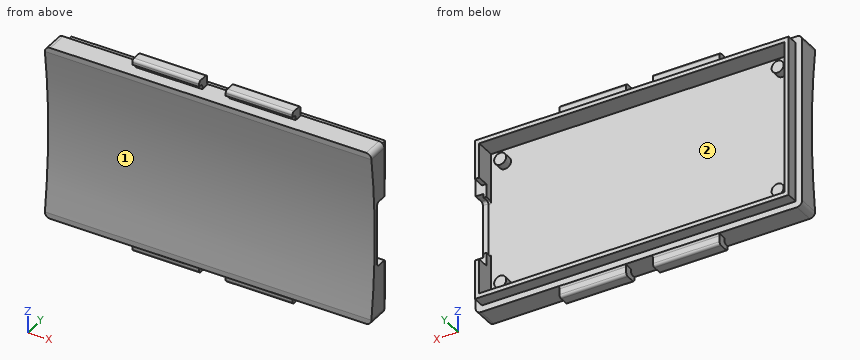
from build123d import *

# Parameters (mm, degrees)
SKETCH2_W               = 61.2
SKETCH2_H               = 32.7
BOSS_EXTRUDE1_DEPTH     = 1.5
BOSS_EXTRUDE2_START     = 1.5
SKETCH2_3_R             = 1.125
BOSS_EXTRUDE2_DEPTH     = 1.5
SKETCH2_7_W             = 61.2
SKETCH2_7_H             = 32.7
BOSS_EXTRUDE5_DEPTH     = 1
FILLET1_R               = 1
CUT_EXTRUDE2_DEPTH      = 35.823591142
CUT_EXTRUDE2_DEPTH_BACK = 0.75
CUT_EXTRUDE2_START      = 1.5
SKETCH2_5_W             = 1.5
SKETCH2_5_H             = 0.75
SKETCH2_5_H_2           = 10.7
FILLET3_R               = 0.5
BOSS_EXTRUDE4_DEPTH     = 2.2
BOSS_EXTRUDE6_DEPTH     = 15
CUT_EXTRUDE4_DEPTH      = 2.5
FILLET4_R               = 0.5
FILLET4_OF_MIRROR1_R    = 0.5
FILLET5_R               = 0.5
CUT_EXTRUDE5_DEPTH      = 37.057211484
CUT_EXTRUDE5_DEPTH_BACK = 37.057211484


with BuildPart() as part:
    # Sketch2 → Boss-Extrude1 (new body)
    with BuildSketch(Plane(origin=(0, 0, 0), x_dir=(1, 0, 0), z_dir=(0, 1, 0))):
        Rectangle(SKETCH2_W, SKETCH2_H)
    extrude(amount=BOSS_EXTRUDE1_DEPTH)

    # Sketch2<3> → Boss-Extrude2 (add)
    with BuildSketch(Plane(origin=(0, 0, 0), x_dir=(1, 0, 0), z_dir=(0, 1, 0)).offset(BOSS_EXTRUDE2_START)):
        Polygon((-30.6, 16.35), (-30.6, -16.35), (30.6, -16.35), (30.6, -6.1), (29.1, -6.1), (29.1, -5.35), (28.6, -5.35), (28.6, -14.35), (-28.6, -14.35), (-28.6, 14.35), (28.6, 14.35), (28.6, 5.35), (30.6, 5.35), (30.6, 16.35), align=None)
        with Locations(Location((-26, 11.75, 0), (0, 0, 270))):
            Circle(SKETCH2_3_R)
        with Locations(Location((-26, -11.75, 0), (0, 0, 270))):
            Circle(SKETCH2_3_R)
        with Locations(Location((26, -11.75, 0), (0, 0, 270))):
            Circle(SKETCH2_3_R)
        with Locations(Location((26, 11.75, 0), (0, 0, 270))):
            Circle(SKETCH2_3_R)
    extrude(amount=BOSS_EXTRUDE2_DEPTH)

    # Sketch2<7> → Boss-Extrude5 (add)
    with BuildSketch(Plane(origin=(0, 0, 0), x_dir=(1, 0, 0), z_dir=(0, 1, 0))):
        Rectangle(SKETCH2_7_W, SKETCH2_7_H)
    extrude(amount=-BOSS_EXTRUDE5_DEPTH)

    # Fillet1
    fillet1_edges = [part.edges().sort_by_distance(p)[0] for p in [
        (-30.6, 1, -16.35),
        (30.6, 1, -16.35),
        (30.6, 1, 16.35),
        (-30.6, 1, 16.35),
    ]]
    fillet(fillet1_edges, radius=FILLET1_R)

    # Sketch2<5> → Cut-Extrude2 (cut, two sides: drawn at the far end of the back side and taken through both)
    with BuildSketch(Plane(origin=(0, 0, 0), x_dir=(1, 0, 0), z_dir=(0, 1, 0)).offset(CUT_EXTRUDE2_START - CUT_EXTRUDE2_DEPTH_BACK)):
        with Locations((29.85, 5.725)):
            Rectangle(SKETCH2_5_W, SKETCH2_5_H)
        with Locations((29.85, 0)):
            Rectangle(SKETCH2_5_W, SKETCH2_5_H_2)
        with Locations((29.85, -5.725)):
            Rectangle(SKETCH2_5_W, SKETCH2_5_H)
    extrude(amount=CUT_EXTRUDE2_DEPTH + CUT_EXTRUDE2_DEPTH_BACK, mode=Mode.SUBTRACT)

    # Fillet3
    fillet3_edges = [part.edges().sort_by_distance(p)[0] for p in [
        (29.85, 0.75, 6.1),
        (29.85, 0.75, -6.1),
        (28.85, 1.5, -5.35),
        (28.85, 1.5, 5.35),
    ]]
    fillet(fillet3_edges, radius=FILLET3_R)

    # Sketch4 → Boss-Extrude4 (add)
    with BuildSketch(Plane(origin=(0, 3, 0), x_dir=(1, 0, 0), z_dir=(0, 1, 0))):
        Polygon((29.4, 15.15), (-29.4, 15.15), (-29.4, -15.15), (29.4, -15.15), (29.4, -7.8), (28.6, -7.8), (28.6, -14.35), (-28.6, -14.35), (-28.6, 14.35), (28.6, 14.35), (28.6, 7.8), (29.4, 7.8), align=None)
    extrude(amount=BOSS_EXTRUDE4_DEPTH)

    # Sketch5 → Boss-Extrude6 (add, symmetric)
    with BuildSketch(Plane(origin=(0, 0, 0), x_dir=(0, 0, -1), z_dir=(1, 0, 0))):
        Polygon((-16.35, 2.8), (-18.35, 2.8), (-18.35, 0.3), (-17.35, 0.3), (-17.35, 1.3), (-16.35, 1.3), align=None)
    boss_extrude6 = extrude(amount=BOSS_EXTRUDE6_DEPTH, both=True)

    # Sketch5<3> → Cut-Extrude4 (cut, symmetric)
    with BuildSketch(Plane(origin=(0, 0, 0), x_dir=(0, 0, -1), z_dir=(1, 0, 0))):
        Polygon((-16.35, 2.8), (-18.35, 2.8), (-18.35, 0.3), (-17.35, 0.3), (-17.35, 1.3), (-16.35, 1.3), align=None)
    cut_extrude4 = extrude(amount=CUT_EXTRUDE4_DEPTH, both=True, mode=Mode.SUBTRACT)

    # Fillet4
    fillet4_edges = [part.edges().sort_by_distance(p)[0] for p in [
        (8.75, 1.3, 17.35),
        (8.75, 2.8, 18.35),
        (8.75, 0.3, 18.35),
        (-8.75, 0.3, 18.35),
        (-8.75, 2.8, 18.35),
        (-8.75, 1.3, 17.35),
    ]]
    fillet(fillet4_edges, radius=FILLET4_R)

    # Mirror1: Boss-Extrude6, Cut-Extrude4 across plane
    add(boss_extrude6.mirror(Plane.XY))
    add(cut_extrude4.mirror(Plane.XY), mode=Mode.SUBTRACT)

    # Fillet4 of Mirror1
    fillet4_of_mirror1_edges = [part.edges().sort_by_distance(p)[0] for p in [
        (8.75, 1.3, -17.35),
        (8.75, 2.8, -18.35),
        (8.75, 0.3, -18.35),
        (-8.75, 0.3, -18.35),
        (-8.75, 2.8, -18.35),
        (-8.75, 1.3, -17.35),
    ]]
    fillet(fillet4_of_mirror1_edges, radius=FILLET4_OF_MIRROR1_R)

    # Fillet5
    # the kernel refuses this fillet: 0.5 mm, written as the material it adds along each edge
    with BuildSketch(Plane(origin=(15, 2.8, 16.35), x_dir=(0, 1.0, 2.6076918401885707e-11), z_dir=(-1, 0, 0)), Plane(origin=(-2.5, 2.8, 16.35), x_dir=(0, 1.0, 2.6076918401885707e-11), z_dir=(-1, 0, 0))) as fillet5_piece_1:
        with BuildLine():
            CenterArc((0.5, -0.4), FILLET5_R, 126.869897647, 53.130102355)
            Line((0, -0.4), (-0.01, -0.4))
            Line((-0.01, -0.4), (-0.01, 0))
            Line((-0.01, 0), (0, 0.01))
            ThreePointArc((0, 0.01), (0.1, 0.01), (0.194, 0.008))
            Line((0.194, 0.008), (0.2, 0))
        make_face()
    extrude(amount=12.5)
    with BuildSketch(Plane(origin=(15, 2.8, -16.35), x_dir=(0, 0, -1), z_dir=(-1, 0, 0))) as fillet5_piece_2:
        with BuildLine():
            CenterArc((0.4, -0.5), FILLET5_R, 90, 53.130102355)
            Line((0, -0.2), (-0.008, -0.194))
            ThreePointArc((-0.008, -0.194), (-0.01, -0.1), (-0.01, 0))
            Line((-0.01, 0), (0, 0.01))
            Line((0, 0.01), (0.4, 0.01))
            Line((0.4, 0.01), (0.4, 0))
        make_face()
    extrude(amount=12.5)
    with BuildSketch(Plane(origin=(-2.5, 2.8, -16.35), x_dir=(0, 1.0, -2.6112445538673017e-11), z_dir=(-1, 0, 0))) as fillet5_piece_3:
        with BuildLine():
            CenterArc((0.5, 0.4), FILLET5_R, 179.999999999, 53.130102355)
            Line((0, 0.4), (-0.01, 0.4))
            Line((-0.01, 0.4), (-0.01, 0))
            Line((-0.01, 0), (0, -0.01))
            ThreePointArc((0, -0.01), (0.1, -0.01), (0.194, -0.008))
            Line((0.194, -0.008), (0.2, 0))
        make_face()
    extrude(amount=12.5)

    # Sketch6 → Cut-Extrude5 (cut, two sides: drawn at the far end of the back side and taken through both)
    with BuildSketch(Plane(origin=(0, 0, 0), x_dir=(0, 0, -1), z_dir=(1, 0, 0)).offset(-CUT_EXTRUDE5_DEPTH_BACK)):
        with BuildLine():
            Line((-15.35, -1), (15.35, -1))
            ThreePointArc((15.35, -1), (0, 0), (-15.35, -1))
        make_face()
    extrude(amount=CUT_EXTRUDE5_DEPTH + CUT_EXTRUDE5_DEPTH_BACK, mode=Mode.SUBTRACT)


solid = part.part
CAD build for the part. Positions are in the model's coordinates, mm. Face numbers are marked on the shaded views. Round coordinates to 2 decimals unless told otherwise and drop trailing zeros. Write each loop counter-clockwise with the first axis right and the second up, starting at its lowest first coordinate (ties: lowest second). Pieces come first, ordered by that corner, then holes.
(1) Probe line 1 along X through (y, z) = (1.75, -11); line 2 along Z through (x, y) = (17.5, 4); line 3 along X through (y, z) = (2.25, -11.5). List the from-to ranges inside material, lowest first.
(2) Drop flat-ended pins along their axis: P1, Ø0.6, axis at x = 5.5, z = -17.5, coming from the -Y side; P2, Ø2.5, axis at x = 26, z = 12, coming from the +Y side; P3, Ø2, axis at y = 1.5, z = -17.5, coming from the -X side. Give the stop position or say it passes through.
(3) Slice it at B-B, the plane x = 18. Write the cut outline in (y, z).
(4) Mould opens along X. For the marked faces 1 and 2 say: pulls with the +X half, pulls with the -X half, needs draft (parallel to the pull), parting line crosses it, or undercut.
(5) Slice it at C-C, the plane z = 0. Write the cut outline in (x, y).
(6) Slice it at A-A, the plane y = 4.5. Write the cut outline in (x, z).
From the geometry:
1. line 1: x = -30.6 to -28.6, -26.84 to -25.16, 25.16 to 26.84, 28.6 to 30.6
1. line 2: z = -15.15 to -14.35, 14.35 to 15.15
1. line 3: x = -30.6 to -28.6, -27.1 to -24.9, 24.9 to 27.1, 28.6 to 30.6
2. P1: stops at y = 0.3
2. P2: stops at y = 3
2. P3: stops at x = -15
3. outline: (-1, -16.35) - (3, -16.35) - (3, -15.15) - (5.2, -15.15) - (5.2, -14.35) - (1.5, -14.35) - (1.5, 14.35) - (5.2, 14.35) - (5.2, 15.15) - (3, 15.15) - (3, 16.35) - (-1, 16.35) - (-1, 15.35) arc R118.31 cw to (-1, -15.35) - close
4. face 1: needs draft
4. face 2: undercut
5. outline: (-30.6, 0) - (30.6, 0) - (30.6, 0.75) - (29.1, 0.75) - (29.1, 1.5) - (-28.6, 1.5) - (-28.6, 5.2) - (-29.4, 5.2) - (-29.4, 3) - (-30.6, 3) - close
6. outline: (-29.4, -15.15) - (29.4, -15.15) - (29.4, -7.8) - (28.6, -7.8) - (28.6, -14.35) - (-28.6, -14.35) - (-28.6, 14.35) - (28.6, 14.35) - (28.6, 7.8) - (29.4, 7.8) - (29.4, 15.15) - (-29.4, 15.15) - close
